For this review, take the finished solid that the model builds, in its own axes (mm). Give positions to 0.01 mm unless a question says otherwise; leave off trailing zeros. Loops run counter-clockwise (first coordinate to the right, second up) from the corner with the lowest first, then second, coordinate; pieces in that order, holes last. Notation, with made-up numbers: (18.25, 48) - (52.25, 48) arc R18 ccw to (52.25, 53) - close; hole circle Ø10 at (48.25, 62). An arc over 180 degrees is marked (long way). Answer in a Markdown table with one row per item.
```python
from build123d import *

# Parameters (mm, degrees)
SKETCH1_W           = 280
SKETCH1_H           = 280
SKETCH1_R           = 16
SKETCH1_R_2         = 7.5
BOSS_EXTRUDE1_DEPTH = 1.5


with BuildPart() as part:
    # Sketch1 → Boss-Extrude1 (new, symmetric)
    with BuildSketch(Plane(origin=(0, 0, 0), x_dir=(1, 0, 0), z_dir=(0, 1, 0))):
        Rectangle(SKETCH1_W, SKETCH1_H)
        with Locations(Location((-104, 96, 0), (0, 0, 270))):
            Circle(SKETCH1_R, mode=Mode.SUBTRACT)
        with Locations(Location((-86.345504448, 10.630092509, 0), (0, 0, 270))):
            Circle(SKETCH1_R_2, mode=Mode.SUBTRACT)
        with Locations(Location((-104, -68.745612269, 0), (0, 0, 270))):
            Circle(SKETCH1_R_2, mode=Mode.SUBTRACT)
        with Locations(Location((36.424311308, -100.557665157, 0), (0, 0, 270))):
            Circle(SKETCH1_R_2, mode=Mode.SUBTRACT)
        with Locations(Location((15.885461628, -8.055627876, 0), (0, 0, 270))):
            Circle(SKETCH1_R_2, mode=Mode.SUBTRACT)
        with Locations(Location((33.226728938, 65.584702367, 0), (0, 0, 270))):
            Circle(SKETCH1_R_2, mode=Mode.SUBTRACT)
        with Locations(Location((102.828111025, 34.411918454, 0), (0, 0, 270))):
            Circle(SKETCH1_R_2, mode=Mode.SUBTRACT)
        with Locations(Location((102.828111025, -70.598741563, 0), (0, 0, 270))):
            Circle(SKETCH1_R_2, mode=Mode.SUBTRACT)
        with Locations(Location((-37.296051937, 63.289287086, 0), (0, 0, 270))):
            Circle(SKETCH1_R_2, mode=Mode.SUBTRACT)
    extrude(amount=BOSS_EXTRUDE1_DEPTH, both=True)


solid = part.part
```
1. We need section A-A, the plane x = -104. Give the boundary of the cut face in (y, z), and give its area (3 significant figures).
Values:
| item | result |
|---|---|
| outline | (-1.5, -140) - (1.5, -140) - (1.5, -112) - (-1.5, -112) - close; (-1.5, -80) - (1.5, -80) - (1.5, 61.25) - (-1.5, 61.25) - close; (-1.5, 76.25) - (1.5, 76.25) - (1.5, 140) - (-1.5, 140) - close |
| area | 699 mm^2 |
2. We need section B-B, the plane z = -96. Give the boundary of the cut face in (x, y).
Values:
| item | result |
|---|---|
| outline | (-140, -1.5) - (-120, -1.5) - (-120, 1.5) - (-140, 1.5) - close; (-88, -1.5) - (140, -1.5) - (140, 1.5) - (-88, 1.5) - close |
3. Wall thickness on line 1 (X direction, y = 1.1, z = -97); line 2 (X direction, y = 0.2, z = 5): over which ranges is each line inside the solid? List them lowest first. Write a range as [from, to].
Values:
| item | result |
|---|---|
| line 1 | x = [-140, -119.97], [-88.03, 140] |
| line 2 | x = [-140, 9.04], [22.73, 140] |
4. We need section C-C, the plane y = -0.45. Count the separate pieces of the cut face and the enclosed holes in it, and give its area (3 significant figures).
Values:
| item | result |
|---|---|
| separate pieces | 1 |
| enclosed holes | 9 |
| area | 76,200 mm^2 |
5. Mouldability with a two-part tool opening along Z and no side actions: class faces 1 (the face through (33.556, -0.021, -73.077)), 2 (the face through (-2, -1.5, -2)) as released by +Z, released by -Z, zero draft, split by the parting line, or undercut.
Values:
| item | result |
|---|---|
| face 1 | undercut |
| face 2 | zero draft |
6. We need section D-D, the plane z = -64. Give the boundary of the cut face in (x, y).
Values:
| item | result |
|---|---|
| outline | (-140, -1.5) - (-44.76, -1.5) - (-44.76, 1.5) - (-140, 1.5) - close; (-29.83, -1.5) - (25.9, -1.5) - (25.9, 1.5) - (-29.83, 1.5) - close; (40.56, -1.5) - (140, -1.5) - (140, 1.5) - (40.56, 1.5) - close |
